Geometry check sheet. Reference: the model listing, model coordinates, mm. A direction names the side the tool comes from. Coordinates: 2 decimals unless noted, no trailing zeros. Write each loop counter-clockwise with the first axis right and the second up, starting at its lowest first coordinate (ties: lowest second). Pieces come first, ordered by that corner, then holes.
from build123d import *

# Parameters (mm, degrees)
F0_R     = 100
F1_DEPTH = 50
F2_R     = 10
F3_W     = 10
F3_H     = 10
F4_DEPTH = 50
F5_W     = 10
F5_H     = 10
F6_DEPTH = 195


with BuildPart() as f1:
    # F0 (on Right) → F1 (new body)
    with BuildSketch(Plane.YZ):
        Circle(F0_R)
    extrude(amount=F1_DEPTH)

    # F2
    f2_edges = [f1.edges().sort_by_distance(p)[0] for p in [
        (50, -100, 0),
        (0, -100, 0),
    ]]
    fillet(f2_edges, radius=F2_R)

    # F3 (on face) → F4 (join)
    with BuildSketch(Plane(origin=(0, 0, 0), x_dir=(0, -1, 0), z_dir=(-1, 0, 0))):
        Rectangle(F3_W, F3_H)
    extrude(amount=F4_DEPTH)

    # F5 (on face) → F6 (join)
    with BuildSketch(Plane.XY.offset(5)):
        with Locations((-45, 0)):
            Rectangle(F5_W, F5_H)
    extrude(amount=F6_DEPTH)


solid = f1.part
1. Sectioned sample at B-B, the plane y = 0. Record the boundary of the cut face in (x, z), and give its area (3 significant figures).
Computed values:
outline: (-50, -5) - (0, -5) - (0, -90) arc R10 ccw to (10, -100) - (40, -100) arc R10 ccw to (50, -90) - (50, 90) arc R10 ccw to (40, 100) - (10, 100) arc R10 ccw to (0, 90) - (0, 5) - (-40, 5) - (-40, 200) - (-50, 200) - close
area: 12,400 mm2
2. Gauge pin test, flat ends, axial feed: pin 1 Ø12 at (y, z) = (-33.5, 99.5) entering from -X; pin 2 Ø1.5 at (x, y) = (36.5, 2) entering from +Z; pin 3 Ø12 at (y, z) = (-79, -54.5) entering from +X; pin 4 Ø3 at (x, y) = (-21, -2) entering from +Z. Record the tip position at first contact, or that the pin passes through.
Computed values:
pin 1: stops at x = 5.62
pin 2: stops at z = 99.99
pin 3: stops at x = 50
pin 4: stops at z = 5
3. Sectioned sample at C-C, the plane x = -28. Record the boundary of the cut face in (y, z), and give its area (3 significant figures).
Computed values:
outline: (-5, -5) - (5, -5) - (5, 5) - (-5, 5) - close
area: 100 mm2
4. Thickness scan on line 1 along X through (y, z) = (23.5, -34.5); line 2 along Y through (x, z) = (15, 12); line 3 along Z through (x, y) = (-27, -4). Record the ranges inside material, lowest first.
Computed values:
line 1: x = 0 to 50
line 2: y = -99.28 to 99.28
line 3: z = -5 to 5
5. Sectioned sample at A-A, the plane z = 0. Record the boundary of the cut face in (x, y), and give its area (3 significant figures).
Computed values:
outline: (-50, -5) - (0, -5) - (0, -90) arc R10 ccw to (10, -100) - (40, -100) arc R10 ccw to (50, -90) - (50, 90) arc R10 ccw to (40, 100) - (10, 100) arc R10 ccw to (0, 90) - (0, 5) - (-50, 5) - close
area: 10,400 mm2
6. Access from +Z, -Z, +X, -X, +Y, -Y to the whole of each face (thin tool, end or side, straight path). Record for faces 1 (the flat face through (-44, 5, 82)), 2 (the flat face through (-25, 0, -5)), 3 (the flat face through (-20, 0, 5)).
Computed values:
face 1: +Z, -Z, -X, +Y
face 2: -Z, -X, +Y, -Y
face 3: +Z, +Y, -Y
7. Sectioned sample at D-D, the plane x = 33.5. Record the boundary of the cut face in (y, z).
Computed values:
outline: circle Ø200 at (0, 0)
8. Draft check along X on faces 4 (the flat face through (-50, 0, 96)), 5 (the flat face through (-40, 0, 101)), 6 (the flat face through (50, -1, 1)), 7 (the flat face through (-44, -5, 82)). Enter one of: released by +X, released by -X, zero draft, split by the parting line, or undercut.
Computed values:
face 4: released by -X
face 5: undercut
face 6: released by +X
face 7: zero draft
